Source: CAD feature listing. Evaluate the final solid. Frame: model axes, mm. Round coordinates to 2 decimals unless told otherwise and drop trailing zeros.
from build123d import *

# Parameters (mm, degrees)
F0_R     = 75
F2_DEPTH = 5
F3_R     = 4.99999
F1_R     = 10
F5_DEPTH = 5


# Not quite as in the source:
# - a fillet or chamfer is up to 0.001 mm smaller than in the source, because OpenCascade refuses the exact size
# - the program builds the solid bodies; features that only make, move or delete a surface that nothing else refers to are left out


with BuildPart() as f2:
    # F0 (on Top) → F2 (new body)
    with BuildSketch(Plane.XY):
        Circle(F0_R)
    extrude(amount=F2_DEPTH)

    # F3 (radius 5 in the source; OpenCascade refuses exactly that, so slightly less here)
    f3_edges = [f2.edges().sort_by_distance(p)[0] for p in [
        (-75, 0, 5),
    ]]
    fillet(f3_edges, radius=F3_R)

    # F1 (on face) → F5 (cut, through all)
    with BuildSketch(Plane.XY):
        with Locations((0, -40)):
            Circle(F1_R)
        with Locations((28.2842712475, -28.2842712475)):
            Circle(F1_R)
        with Locations((-28.2842712475, -28.2842712475)):
            Circle(F1_R)
        with Locations((-40, 0)):
            Circle(F1_R)
        with Locations((-28.2842712475, 28.2842712475)):
            Circle(F1_R)
        with Locations((0, 40)):
            Circle(F1_R)
        with Locations((28.2842712475, 28.2842712475)):
            Circle(F1_R)
        with Locations((40, 0)):
            Circle(F1_R)
    extrude(amount=F5_DEPTH, mode=Mode.SUBTRACT)


solid = f2.part
1) Section query A-A on y = 0. State how many separate pieces and enclosed holes the cut face has, then the cut area to 3 significant figures.
Taken from the geometry:
separate pieces: 3
enclosed holes: 0
area: 539 mm2
2) Material intervals for line 1 (X direction, y = -25.5, z = 0.6); line 2 (Y direction, x = 0, z = 3.1); line 3 (Y direction, x = 0, z = 1.85), sorted ascending.
Taken from the geometry:
line 1: x = -70.49 to -37.89, -18.68 to 18.68, 37.89 to 70.49
line 2: y = -73.92 to -50, -30 to 30, 50 to 73.92
line 3: y = -74.65 to -50, -30 to 30, 50 to 74.65
3) Contact query for flat-ended pins moving along their axis: P1, Ø3, axis at y = -24.5, z = 3.5, coming from the -X side; P2, Ø2, axis at x = -14, z = 3.5, coming from the +Y side. Output: stop coordinate, or through.
Taken from the geometry:
P1: stops at x = -70.6
P2: stops at y = 73.03
4) Pull-direction query (Y, two-part tool) for faces 1 (the face through (-2.17, -49.76, 2.46)), 2 (the face through (18.294, -27.845, 2.465)), 3 (the face through (-1, 1, 5)); classes: released by +Y, released by -Y, zero draft, split by the parting line, or undercut.
Taken from the geometry:
face 1: undercut
face 2: undercut
face 3: zero draft
